Here's how the part is built. I have some questions about the finished solid (model axes, mm). Coordinates: 2 decimals unless noted, no trailing zeros. Write each loop counter-clockwise with the first axis right and the second up, starting at its lowest first coordinate (ties: lowest second). Pieces come first, ordered by that corner, then holes.
Item 1: I'm going to push a flat-ended pin straight in: P1, Ø6.5, axis at x = -175, y = 175, coming from the +Z side. Where does the tip first touch, or does it pass through?
Item 2: I want a section at B-B (x = 14). Please give me the cut outline in (y, z), and give its area (3 significant figures).
Item 3: Please list where these lines run through material, in increasing order: line 1 (Y direction, x = 175, z = 2.9); line 2 (X direction, y = -152.5, z = 1.05); line 3 (Y direction, x = 62.5, z = 1.5).
Item 4: I want a section at A-A (y = 25.5). Please give me the cut outline in (x, z), and give its area (3 significant figures).
Item 5: I want a section at C-C (z = 2.6). Count the separate pieces of the cut face and the enclosed holes in it, and give its area (3 significant figures).
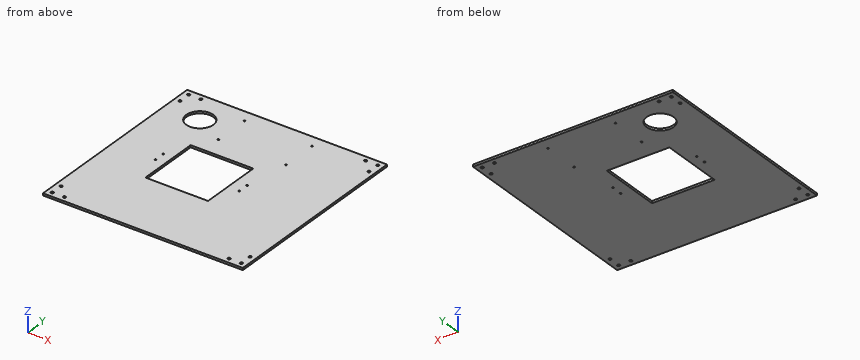
from build123d import *

# Parameters (mm, degrees)
SKETCH_1_W          = 370
SKETCH_1_H          = 370
EXTRUDE_1_DEPTH     = 4
SKETCH_2_R          = 2.5
CUT_EXTRUDE_1_DEPTH = 262.660084843
SKETCH_4_W          = 116
SKETCH_4_H          = 116
CUT_EXTRUDE_5_DEPTH = 262.660084843
SKETCH_6_R          = 1.5
CUT_EXTRUDE_7_DEPTH = 262.660084843
SKETCH_7_R          = 25
CUT_EXTRUDE_8_DEPTH = 262.660084843
SKETCH_8_R          = 1.5
CUT_EXTRUDE_9_DEPTH = 10


with BuildPart() as part:
    # 草图1 → 凸台-拉伸1 (new body)
    with BuildSketch(Plane.XY):
        Rectangle(SKETCH_1_W, SKETCH_1_H)
    extrude(amount=EXTRUDE_1_DEPTH)

    # 草图2 → 切除-拉伸1 (cut, through all)
    with BuildSketch(Plane.XY.offset(4)):
        with Locations((-175, -175)):
            Circle(SKETCH_2_R)
        with Locations((-152.5, -175)):
            Circle(SKETCH_2_R)
        with Locations((-175, -152.5)):
            Circle(SKETCH_2_R)
        with Locations((-152.5, 175)):
            Circle(SKETCH_2_R)
        with Locations((-175, 152.5)):
            Circle(SKETCH_2_R)
        with Locations((-175, 175)):
            Circle(SKETCH_2_R)
        with Locations((175, 152.5)):
            Circle(SKETCH_2_R)
        with Locations((152.5, 175)):
            Circle(SKETCH_2_R)
        with Locations((175, 175)):
            Circle(SKETCH_2_R)
        with Locations((152.5, -175)):
            Circle(SKETCH_2_R)
        with Locations((175, -152.5)):
            Circle(SKETCH_2_R)
        with Locations((175, -175)):
            Circle(SKETCH_2_R)
    extrude(amount=-CUT_EXTRUDE_1_DEPTH, mode=Mode.SUBTRACT)

    # 草图4 → 切除-拉伸5 (cut, through all)
    with BuildSketch(Plane(origin=(0, 0, 0), x_dir=(-1, 0, 0), z_dir=(0, 0, -1))):
        with Locations((28.956152895, -0.09)):
            Rectangle(SKETCH_4_W, SKETCH_4_H)
    extrude(amount=-CUT_EXTRUDE_5_DEPTH, mode=Mode.SUBTRACT)

    # 草图6 → 切除-拉伸7 (cut, through all)
    with BuildSketch(Plane(origin=(0, 0, 0), x_dir=(-1, 0, 0), z_dir=(0, 0, -1))):
        with Locations((-62.5, 162.249795252)):
            Circle(SKETCH_6_R)
        with Locations((-62.5, 95.249795252)):
            Circle(SKETCH_6_R)
        with Locations((62.5, 95.249795252)):
            Circle(SKETCH_6_R)
        with Locations((62.5, 162.249795252)):
            Circle(SKETCH_6_R)
    extrude(amount=-CUT_EXTRUDE_7_DEPTH, mode=Mode.SUBTRACT)

    # 草图7 → 切除-拉伸8 (cut, through all)
    with BuildSketch(Plane(origin=(0, 0, 0), x_dir=(-1, 0, 0), z_dir=(0, 0, -1))):
        with Locations((118.769854949, 125.631801741)):
            Circle(SKETCH_7_R)
    extrude(amount=-CUT_EXTRUDE_8_DEPTH, mode=Mode.SUBTRACT)

    # 草图8 → 切除-拉伸9 (cut)
    with BuildSketch(Plane(origin=(0, 0, 0), x_dir=(-1, 0, 0), z_dir=(0, 0, -1))):
        with Locations((-50.21335715, -7.305969028)):
            Circle(SKETCH_8_R)
        with Locations((-50.21335715, 12.694030972)):
            Circle(SKETCH_8_R)
        with Locations((104.956152895, -7.308718804)):
            Circle(SKETCH_8_R)
        with Locations((104.956152895, 12.691281196)):
            Circle(SKETCH_8_R)
    extrude(amount=-CUT_EXTRUDE_9_DEPTH, mode=Mode.SUBTRACT)


solid = part.part
Answer:
1. P1: stops at z = 4
2. outline: (-185, 0) - (-58.09, 0) - (-58.09, 4) - (-185, 4) - close; (57.91, 0) - (185, 0) - (185, 4) - (57.91, 4) - close
2. area: 1,020 mm2
3. line 1: y = -185 to -177.5, -172.5 to -155, -150 to 150, 155 to 172.5, 177.5 to 185
3. line 2: x = -185 to -177.5, -172.5 to 172.5, 177.5 to 185
3. line 3: y = -185 to 93.75, 96.75 to 160.75, 163.75 to 185
4. outline: (-185, 0) - (-86.96, 0) - (-86.96, 4) - (-185, 4) - close; (29.04, 0) - (185, 0) - (185, 4) - (29.04, 4) - close
4. area: 1,020 mm2
5. separate pieces: 1
5. enclosed holes: 22
5. area: 121,000 mm2
